Autodesk Inventor part; units mm, degrees
ref_plane "YZ Plane" through (0, 0, 0) normal (1, 0, 0) x (0, 1, 0)
ref_plane "XZ Plane" through (0, 0, 0) normal (0, 1, 0) x (-1, 0, 0)
ref_plane "XY Plane" through (0, 0, 0) normal (0, 0, 1) x (1, 0, 0)
sketch "Sketch1" plane through (0, 0, 0) normal (0, 1, 0) x (-1, 0, 0)
  line L0 (0, 0) -> (25, 0)
  line L1 (25, 0) -> (25, -50)
  line L2 (25, -50) -> (0, -50)
  line L3 (0, -50) -> (0, 0)
  dimension "d0" = 25
  dimension "d1" = 50
extrude "Extrusion1" add sketch "Sketch1" along normal blind 5
sketch "Sketch2" plane through (0, 5, 0) normal (0, 1, 0) x (1, 0, 0)
  point P0 (0, 0)
sketch "Sketch3" plane through (0, 5, 0) normal (0, 1, 0) x (1, 0, 0)
  circle A0 centre (-21.608, 3) radius 1
  circle A1 centre (-21.608, 47) radius 1
  line L0 (-25, 0) -> (0, 0)
  dimension "d4" = 2
  dimension "d5" = 2
  dimension "d6" = 44
  dimension "d7" = 3
extrude "Extrusion2" cut sketch "Sketch3" against normal through all
sketch "Sketch4" plane through (0, 5, 0) normal (0, 1, 0) x (1, 0, 0)
  circle A0 centre (-5, 3) radius 1.5
  circle A1 centre (-5, 47) radius 1.5
  point P0 (0, 0)
  dimension "d10" = 3
  dimension "d11" = 3
extrude "Extrusion3" cut sketch "Sketch4" against normal blind 10
properties part number "ULTREALJUD"
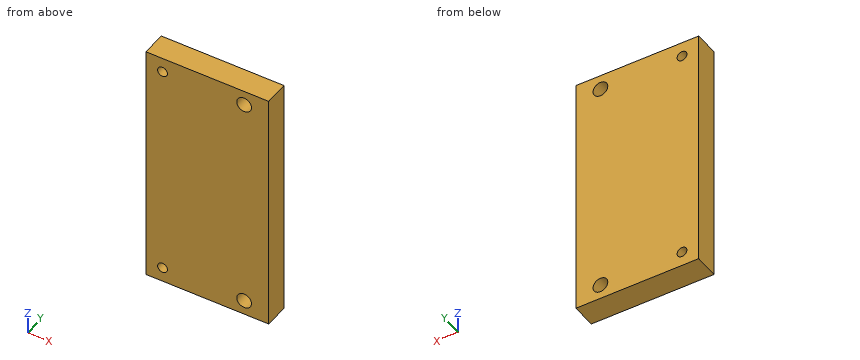
Check sheet for the modelled part. Datum: model origin and axes. Units: mm. Coordinates: 2 decimals unless noted, no trailing zeros. Loops run counter-clockwise (first coordinate to the right, second up) from the corner with the lowest first, then second, coordinate; pieces in that order, holes last.
1) Material ranges on probe 1 along X at (y, z) = (2.9, -3); probe 2 along Z at (x, y) = (-5, 2.6); probe 3 along Z at (x, y) = (-5.5, 3.1), recorded low to high.
2) Sectioned sample at C-C (y = 1.7). Record the boundary of the cut face in (x, z), and give its area (3 significant figures).
3) Sectioned sample at B-B (z = -3). Record the boundary of the cut face in (x, y), and give its area (3 significant figures).
4) Sectioned sample at A-A (x = -5). Record the boundary of the cut face in (y, z).
Check sheet entries:
1. probe 1: x = -25 to -22.61, -20.61 to -6.5, -3.5 to 0
1. probe 2: z = -50 to -48.5, -45.5 to -4.5, -1.5 to 0
1. probe 3: z = -50 to -48.41, -45.59 to -4.41, -1.59 to 0
2. outline: (-25, -50) - (0, -50) - (0, 0) - (-25, 0) - close; hole circle Ø2 at (-21.61, -47); hole circle Ø2 at (-21.61, -3); hole circle Ø3 at (-5, -47); hole circle Ø3 at (-5, -3)
2. area: 1,230 mm2
3. outline: (-25, 0) - (-22.61, 0) - (-22.61, 5) - (-25, 5) - close; (-20.61, 0) - (-6.5, 0) - (-6.5, 5) - (-20.61, 5) - close; (-3.5, 0) - (0, 0) - (0, 5) - (-3.5, 5) - close
3. area: 100 mm2
4. outline: (0, -50) - (5, -50) - (5, -48.5) - (0, -48.5) - close; (0, -45.5) - (5, -45.5) - (5, -4.5) - (0, -4.5) - close; (0, -1.5) - (5, -1.5) - (5, 0) - (0, 0) - close
